The listing builds one solid part. Answer for the finished solid, in the listing's coordinates (mm). A direction names the side the tool comes from. Give positions to 0.01 mm unless a question says otherwise; leave off trailing zeros. Order: outer loops, then holes, each group sorted by start corner. A loop starts at its lowest first (then second) coordinate and runs counter-clockwise, first axis right, second up. Notation, with made-up numbers: (40, 34.25) - (55, 34.25) arc R7 cw to (55, 45.25) - close; hole circle Ø7 at (-13, 60.5). An arc over 180 degrees is marked (long way). Answer as CSV lines item,"result". Start each with the question number.
1. Section B-B on x = 10.25 is taken. Give the vertices of the cut face in (y, z), and give its area (3 significant figures).
2. Which of the six approach directions +Z, -Z, +X, -X, +Y, -Y give full straight-line access (tool end or side, diameter ignored) to faces 5 (the flat face through (3, -81.12, 5)), 6 (the cylindrical face through (3.21, -78.55, 2.12)), 7 (the flat face through (3, -86, 10))?
3. Section A-A on y = -80.25 is taken. Give the vertices of the cut face in (x, z), and give its area (3 significant figures).
4. Flat-ended cylindrical pins translate along their axes: pin 1 (1.5 mm diameter, centred on x = 4, y = -87, fed in from -Z); pin 2 (5.5 mm diameter, centred on x = 3.5, y = -74.5, fed in from -Z). Find the tip coordinate at first contact, or state that the pin passes through.
5. Section D-D on x = 2.25 is taken. Give the vertices of the cut face in (y, z), and give its area (3 significant figures).
6. Section C-C on z = 6.5 is taken. Give the vertices of the cut face in (x, y).
7. Determine the mould class of faces 1 (the flat face through (3, -101.05, 5)), 2 (the flat face through (-3.2, -79.3, 3.5)), 3 (the flat face through (3, -75, 1.52)), 4 (the cylindrical face through (-6.1, -89.57, 5.07)) for opening direction Y: +Y half, -Y half, draft (parallel to the pull), parting line (faces both ways), or undercut.
8. Consider line 1 along Y through (x, z) = (-2.5, 9.25); line 2 along Y through (x, z) = (-2.5, 1.75); line 3 along X through (y, z) = (-79.5, 4.75). Determine where each line is inside the solid, lowest interval first. Write a range as [from, to].
from build123d import *

# Parameters (mm, degrees)
SKETCH1_W           = 30
SKETCH1_H           = 28.98
SKETCH1_W_2         = 13
SKETCH1_H_2         = 2
SKETCH1_W_3         = 20
SKETCH1_H_3         = 5
BOSS_EXTRUDE1_DEPTH = 10
FILLET1_R           = 2
SKETCH2_W           = 13
SKETCH2_H           = 7.05
CUT_EXTRUDE1_DEPTH  = 1.52
FILLET2_R           = 2


with BuildPart() as part:
    # Sketch1 → Boss-Extrude1 (new body)
    with BuildSketch(Plane.XY):
        with Locations((3.3, -86.56)):
            Rectangle(SKETCH1_W, SKETCH1_H)
        with Locations((3.3, -80.12)):
            Rectangle(SKETCH1_W_2, SKETCH1_H_2, mode=Mode.SUBTRACT)
        with Locations((3.3, -91.5)):
            Rectangle(SKETCH1_W_3, SKETCH1_H_3, mode=Mode.SUBTRACT)
    extrude(amount=BOSS_EXTRUDE1_DEPTH)

    # Fillet1
    fillet1_edges = [part.edges().sort_by_distance(p)[0] for p in [
        (-6.7, -89, 5),
        (-6.7, -94, 5),
        (13.3, -94, 5),
        (13.3, -89, 5),
    ]]
    fillet(fillet1_edges, radius=FILLET1_R)

    # Sketch2 → Cut-Extrude1 (cut)
    with BuildSketch(Plane(origin=(0, 0, 0), x_dir=(-1, 0, 0), z_dir=(0, 0, -1))):
        with Locations((-3.3, -75.595)):
            Rectangle(SKETCH2_W, SKETCH2_H)
    extrude(amount=-CUT_EXTRUDE1_DEPTH, mode=Mode.SUBTRACT)

    # Fillet2
    fillet2_edges = [part.edges().sort_by_distance(p)[0] for p in [
        (3.3, -79.12, 1.52),
    ]]
    fillet(fillet2_edges, radius=FILLET2_R)


solid = part.part
Checks:
1,outline,"(-101.05, 0) - (-94, 0) - (-94, 10) - (-101.05, 10) - close; (-89, 0) - (-72.07, 0) - (-72.07, 10) - (-89, 10) - close"
1,area,"240 mm²"
2,face 5,"+Z, -Z"
2,face 6,"-Z"
2,face 7,"+Z, +X, -X, +Y, -Y"
3,outline,"(-11.7, 0) - (-3.2, 0) - (-3.2, 10) - (-11.7, 10) - close; (9.8, 0) - (18.3, 0) - (18.3, 10) - (9.8, 10) - close"
3,area,"170 mm²"
4,pin 1,"stops at z = 0"
4,pin 2,"stops at z = 1.52"
5,outline,"(-101.05, 0) - (-94, 0) - (-94, 10) - (-101.05, 10) - close; (-89, 0) - (-81.12, 0) - (-81.12, 10) - (-89, 10) - close; (-79.12, 3.52) arc R2 ccw to (-77.12, 1.52) - (-72.07, 1.52) - (-72.07, 10) - (-79.12, 10) - close"
5,area,"208 mm²"
6,outline,"(-11.7, -101.05) - (18.3, -101.05) - (18.3, -72.07) - (-11.7, -72.07) - close; hole (-6.7, -92) arc R2 ccw to (-4.7, -94) - (11.3, -94) arc R2 ccw to (13.3, -92) - (13.3, -91) arc R2 ccw to (11.3, -89) - (-4.7, -89) arc R2 ccw to (-6.7, -91) - close; hole (-3.2, -81.12) - (9.8, -81.12) - (9.8, -79.12) - (-3.2, -79.12) - close"
7,face 1,"-Y half"
7,face 2,"undercut"
7,face 3,"draft"
7,face 4,"undercut"
8,line 1,"y = [-101.05, -94], [-89, -81.12], [-79.12, -72.07]"
8,line 2,"y = [-101.05, -94], [-89, -81.12], [-78.05, -72.07]"
8,line 3,"x = [-11.7, -3.2], [9.8, 18.3]"
